Geometry check sheet. Reference: drawing and pictorial views, mm from the part's lowest x, y, z. Give positions to 0.01 mm unless a question says otherwise; leave off trailing zeros. Order: outer loops, then holes, each group sorted by start corner. A loop starts at its lowest first (then second) coordinate and runs counter-clockwise, first axis right, second up. Notation, with made-up numbers: (13.5, 15.5) - (45.5, 15.5) arc R22 ccw to (45.5, 47.5) - close; hole circle Ø6 at (63.5, -6). An arc over 180 degrees is marked (long way). Answer as a JSON object with one key per item and string values.
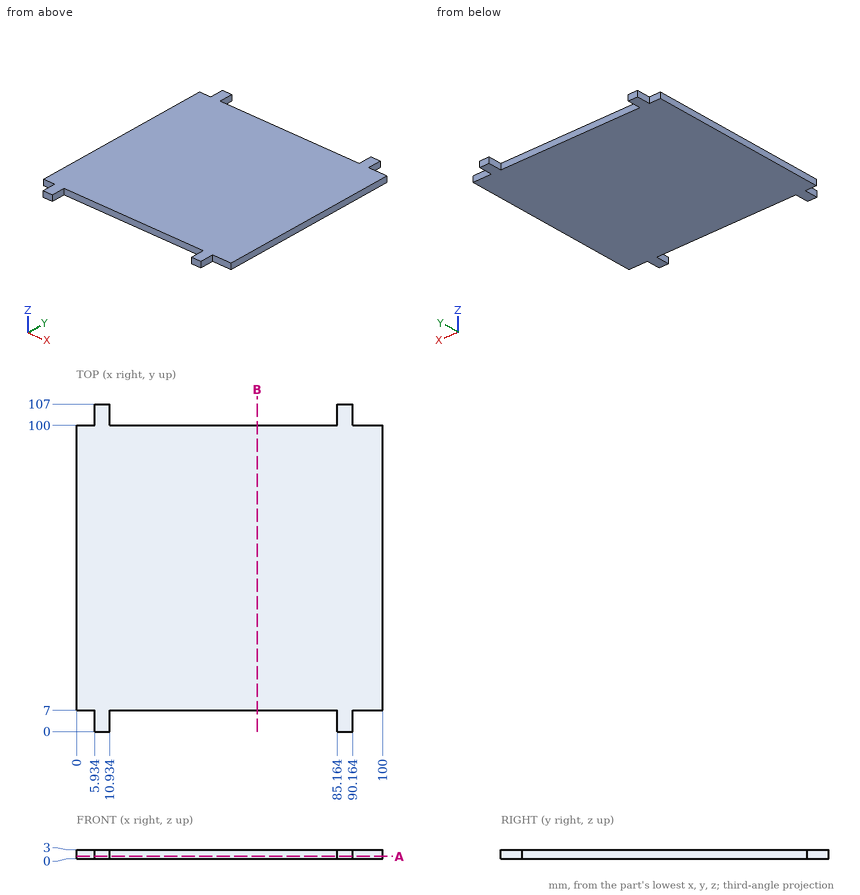
(1) Material ranges on line 1 along X through (y, z) = (102, 2.55); line 2 along Y through (x, z) = (24.5, 0.95), recorded low to high. Write a range as [from, to].
Computed values:
{"line 1": "x = [5.93, 10.93], [85.16, 90.16]", "line 2": "y = [7, 100]"}
(2) Section check B-B (x = 59). Record the cut outline in (y, z).
Computed values:
{"outline": "(7, 0) - (100, 0) - (100, 3) - (7, 3) - close"}
(3) Gauge pin test, flat ends, axial feed: pin 1 Ø0.9 at (x, z) = (31, 1) entering from -Y; pin 2 Ø1.5 at (y, z) = (103.5, 1.5) entering from -X; pin 3 Ø0.9 at (y, z) = (102, 1.5) entering from +X. Record the tip position at first contact, or that the pin passes through.
Computed values:
{"pin 1": "stops at y = 7", "pin 2": "stops at x = 5.93", "pin 3": "stops at x = 90.16"}
(4) Section check A-A (z = 0.8). Record the cut outline in (x, y), then the cut area to 3 significant figures.
Computed values:
{"outline": "(0, 7) - (5.93, 7) - (5.93, 0) - (10.93, 0) - (10.93, 7) - (85.16, 7) - (85.16, 0) - (90.16, 0) - (90.16, 7) - (100, 7) - (100, 100) - (90.16, 100) - (90.16, 107) - (85.16, 107) - (85.16, 100) - (10.93, 100) - (10.93, 107) - (5.93, 107) - (5.93, 100) - (0, 100) - close", "area": "9,440 mm²"}
